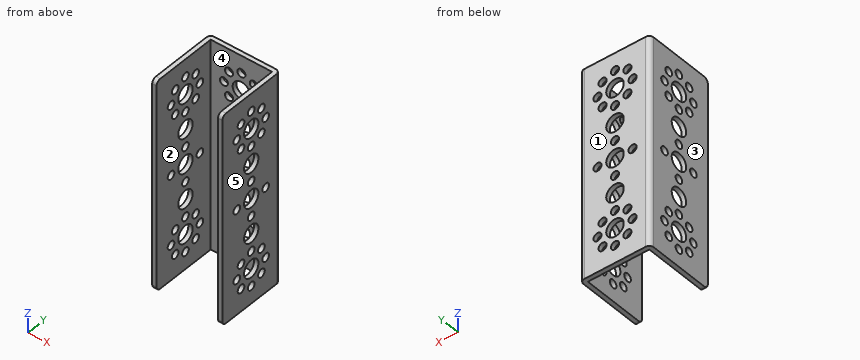
```python
from build123d import *

# Parameters (mm, degrees)
BOSS_EXTRUDE1_DEPTH = 96
SKETCH2_R           = 4
SKETCH2_R_2         = 1.85
CUT_EXTRUDE1_DEPTH  = 33
SKETCH3_R           = 4
SKETCH3_R_2         = 1.85
CUT_EXTRUDE2_DEPTH  = 33
FILLET1_R           = 2


with BuildPart() as part:
    # Sketch1 → Boss-Extrude1 (new body)
    with BuildSketch(Plane.XY):
        Polygon((14, -16), (16, -16), (16, 16), (-16, 16), (-16, -16), (-14, -16), (-14, 14), (14, 14), align=None)
    extrude(amount=-BOSS_EXTRUDE1_DEPTH)

    # Sketch2 → Cut-Extrude1 (cut, through all)
    with BuildSketch(Plane(origin=(0, 16, 0), x_dir=(1, 0, 0), z_dir=(0, 1, 0))):
        with Locations((0, 32)):
            Circle(SKETCH2_R)
        with Locations((0, 64)):
            Circle(SKETCH2_R)
        with Locations((0, 48)):
            Circle(SKETCH2_R)
        with Locations((0, 56)):
            Circle(SKETCH2_R_2)
        with Locations((0, 40)):
            Circle(SKETCH2_R_2)
        with Locations((8, 48)):
            Circle(SKETCH2_R_2)
        with Locations((-8, 48)):
            Circle(SKETCH2_R_2)
        with Locations((0, 24)):
            Circle(SKETCH2_R_2)
        with Locations((8, 16)):
            Circle(SKETCH2_R_2)
        with Locations((0, 16)):
            Circle(SKETCH2_R)
        with Locations((-8, 16)):
            Circle(SKETCH2_R_2)
        with Locations((-5.66, 10.34)):
            Circle(SKETCH2_R_2)
        with Locations((5.66, 10.34)):
            Circle(SKETCH2_R_2)
        with Locations((0, 8)):
            Circle(SKETCH2_R_2)
        with Locations((-5.66, 21.66)):
            Circle(SKETCH2_R_2)
        with Locations((5.66, 21.66)):
            Circle(SKETCH2_R_2)
        with Locations((0, 88)):
            Circle(SKETCH2_R_2)
        with Locations((8, 80)):
            Circle(SKETCH2_R_2)
        with Locations((0, 80)):
            Circle(SKETCH2_R)
        with Locations((-8, 80)):
            Circle(SKETCH2_R_2)
        with Locations((-5.66, 74.34)):
            Circle(SKETCH2_R_2)
        with Locations((5.66, 74.34)):
            Circle(SKETCH2_R_2)
        with Locations((0, 72)):
            Circle(SKETCH2_R_2)
        with Locations((-5.66, 85.66)):
            Circle(SKETCH2_R_2)
        with Locations((5.66, 85.66)):
            Circle(SKETCH2_R_2)
    extrude(amount=-CUT_EXTRUDE1_DEPTH, mode=Mode.SUBTRACT)

    # Sketch3 → Cut-Extrude2 (cut, through all)
    with BuildSketch(Plane(origin=(16, 0, 0), x_dir=(0, 0, -1), z_dir=(1, 0, 0))):
        with Locations((64, 0)):
            Circle(SKETCH3_R)
        with Locations((32, 0)):
            Circle(SKETCH3_R)
        with Locations((48, 0)):
            Circle(SKETCH3_R)
        with Locations((40, 0)):
            Circle(SKETCH3_R_2)
        with Locations((56, 0)):
            Circle(SKETCH3_R_2)
        with Locations((48, 8)):
            Circle(SKETCH3_R_2)
        with Locations((48, -8)):
            Circle(SKETCH3_R_2)
        with Locations((72, 0)):
            Circle(SKETCH3_R_2)
        with Locations((80, 8)):
            Circle(SKETCH3_R_2)
        with Locations((80, 0)):
            Circle(SKETCH3_R)
        with Locations((80, -8)):
            Circle(SKETCH3_R_2)
        with Locations((85.66, -5.66)):
            Circle(SKETCH3_R_2)
        with Locations((85.66, 5.66)):
            Circle(SKETCH3_R_2)
        with Locations((88, 0)):
            Circle(SKETCH3_R_2)
        with Locations((74.34, -5.66)):
            Circle(SKETCH3_R_2)
        with Locations((74.34, 5.66)):
            Circle(SKETCH3_R_2)
        with Locations((8, 0)):
            Circle(SKETCH3_R_2)
        with Locations((16, 8)):
            Circle(SKETCH3_R_2)
        with Locations((16, 0)):
            Circle(SKETCH3_R)
        with Locations((16, -8)):
            Circle(SKETCH3_R_2)
        with Locations((21.66, -5.66)):
            Circle(SKETCH3_R_2)
        with Locations((21.66, 5.66)):
            Circle(SKETCH3_R_2)
        with Locations((24, 0)):
            Circle(SKETCH3_R_2)
        with Locations((10.34, -5.66)):
            Circle(SKETCH3_R_2)
        with Locations((10.34, 5.66)):
            Circle(SKETCH3_R_2)
    extrude(amount=-CUT_EXTRUDE2_DEPTH, mode=Mode.SUBTRACT)

    # Fillet1
    fillet1_edges = [part.edges().sort_by_distance(p)[0] for p in [
        (-15, -16, -96),
        (-16, 16, -48),
        (16, 16, -48),
        (15, -16, -96),
        (15, -16, 0),
        (-15, -16, 0),
    ]]
    fillet(fillet1_edges, radius=FILLET1_R)


solid = part.part
```
CAD build for the part. Positions are in the model's coordinates, mm. Face numbers are marked on the shaded views. A direction names the side the tool comes from. Round coordinates to 2 decimals unless told otherwise and drop trailing zeros. Order: outer loops, then holes, each group sorted by start corner. A loop starts at its lowest first (then second) coordinate and runs counter-clockwise, first axis right, second up. Notation, with made-up numbers: (40.25, 19) -> (89.25, 19) arc R21 ccw to (89.25, 53) -> close; hole circle Ø2 at (-6, 8.5). An arc over 180 degrees is marked (long way). Write item = value, one per line.
(1) Flat gauge pins, fed straight in: P1, Ø3.5, axis at x = 0, z = -8, coming from the -Y side; P2, Ø2, axis at x = 9.5, z = -32.5, coming from the -Y side. Where does each tip first touch, or does it go through?
Answers follow:
P1 = through
P2 = 14
(2) Pull direction X, two halves, no side cores. Call the marked faces 1, 2 and 3: +X half, -X half, draft (parallel to the pull), parting line (faces both ways), or undercut.
Answers follow:
face_1 = draft
face_2 = undercut
face_3 = -X half
(3) Cut at B-B (y = 9). State how many separate pieces and enclosed holes the cut face has, plus the area to 3 significant figures.
Answers follow:
separate_pieces = 8
enclosed_holes = 0
area = 347 mm²
(4) 3-axis set-ups, long thin cutter, end or side, ignore diameter. For the marked faces 4 and 5: which of +Z, -Z, +X, -X, +Y, -Y reach the whole face in a straight line?
Answers follow:
face_4 = +Z, -Z, -Y
face_5 = +Z, -Z, +X, +Y, -Y
(5) Cut at A-A (z = -64). Write the cut outline in (x, y).
Answers follow:
outline = (-16, -16) -> (-14, -16) -> (-14, -4) -> (-16, -4) -> close; (-16, 4) -> (-14, 4) -> (-14, 14) -> (-4, 14) -> (-4, 16) -> (-14, 16) arc R2 ccw to (-16, 14) -> close; (4, 14) -> (14, 14) -> (14, 4) -> (16, 4) -> (16, 14) arc R2 ccw to (14, 16) -> (4, 16) -> close; (14, -16) -> (16, -16) -> (16, -4) -> (14, -4) -> close
(6) Drill centre lines: L1, parallel to X at y = -3.5, z = -73; L2, parallel to Y at x = -15.45, z = -74.34; L3, parallel to Y at x = 10, z = -13. Where is each one in solid material? Low to high.
Answers follow:
L1 = -16 to -14, 14 to 16
L2 = -16 to -7.51, -3.81 to 3.81, 7.51 to 15.38
L3 = 14 to 16
